Verification items for this drawing (mm, ordinates from the low corner). A direction names the side the tool comes from. Coordinates: 2 decimals unless noted, no trailing zeros. Order: outer loops, then holes, each group sorted by start corner. A loop starts at its lowest first (then second) coordinate and runs counter-clockwise, first axis right, second up. Notation, with made-up numbers: M 10,-25.5 L 22,-25.5 A7 ccw 22,-16.5 Z; hole C 60,55 d1. An arc over 180 degrees is marked long. Answer as a JSON object with one key per item and string values. Group by question number.
(1) Gauge pin test, flat ends, axial feed: pin 1 Ø5 at (y, z) = (11.5, 11.5) entering from -X; pin 2 Ø5 at (y, z) = (7.5, 28) entering from -X; pin 3 Ø3 at (y, z) = (9, 8.5) entering from +X; pin 4 Ø10 at (y, z) = (11.5, 12) entering from +X. Record the tip position at first contact, or that the pin passes through.
(2) Cross-section at D-D (z = 9.5). Enter the section's corners in (x, y), plus the area to 3 significant figures.
(3) Cross-section at C-C (x = 23). Enter the section's corners in (y, z), plus the area to 3 significant figures.
(4) Material ranges on line 1 (Z direction, x = 47, y = 4.75); line 2 (Z direction, x = 56.5, y = 14); line 3 (X direction, y = 1.75, z = 27.5) (1 decimal), recorded low to high.
(5) Access from +Z, -Z, +X, -X, +Y, -Y to the whole of each face (thin tool, end or side, straight path). Record for the marked faces 1, 2 and 3.
(6) Cross-section at B-B (y = 9.5). Enter the section's corners in (x, z), plus the area to 3 significant figures.
(7) Cross-section at A-A (x = 62). Enter the section's corners in (y, z).
(8) Mould release check, pull along Z, two halves, no side actions. Record for the marked faces 4, 5, 6 and 7: released by +Z, released by -Z, zero draft, split by the parting line, or undercut.
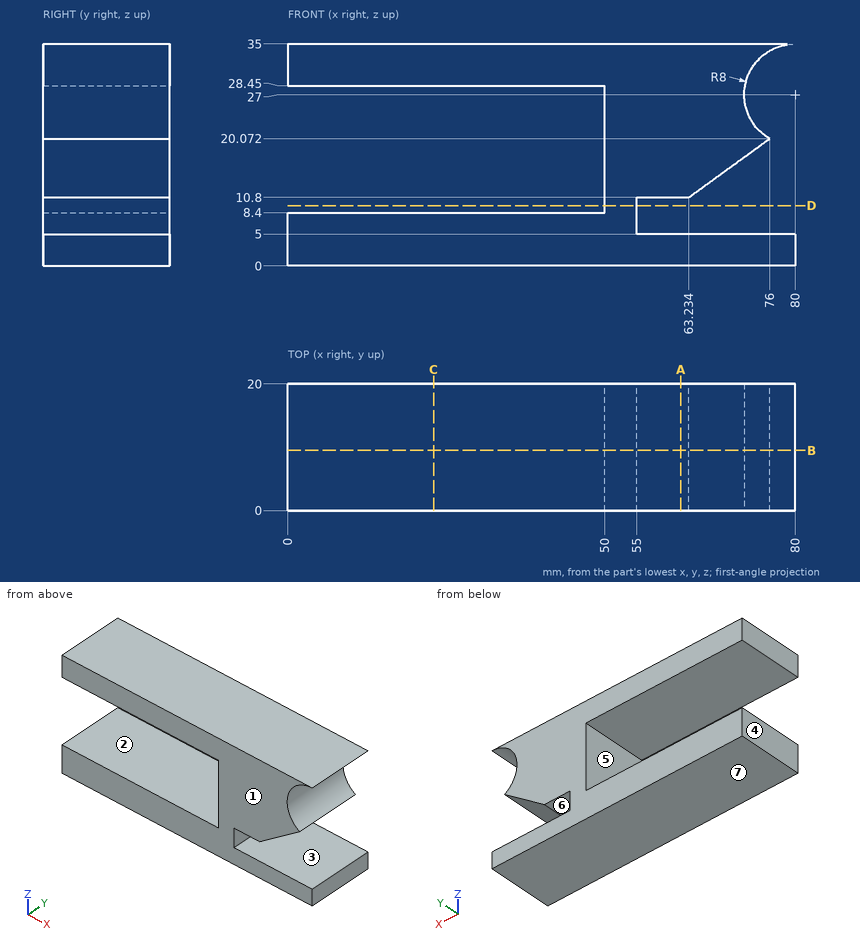
Taken from the geometry:
{
 "1": {"pin 1": "stops at x = 50", "pin 2": "stops at x = 0", "pin 3": "stops at x = 55", "pin 4": "stops at x = 71.77"},
 "2": {"outline": "M 50,0 L 55,0 L 55,20 L 50,20 Z", "area": "100 mm²"},
 "3": {"outline": "M 0,0 L 20,0 L 20,8.4 L 0,8.4 Z; M 0,28.45 L 20,28.45 L 20,35 L 0,35 Z", "area": "299 mm²"},
 "4": {"line 1": "z = 0 to 8.4, 28.45 to 35", "line 2": "z = 0 to 5, 10.8 to 35", "line 3": "x = 50 to 72"},
 "5": {"face 1": "+Z, -Z, +X, -X, -Y", "face 2": "-X, +Y, -Y", "face 3": "+X, +Y, -Y"},
 "6": {"outline": "M 0,0 L 80,0 L 80,5 L 55,5 L 55,10.8 L 63.23,10.8 L 76,20.07 A8 cw 80,35 L 0,35 L 0,28.45 L 50,28.45 L 50,8.4 L 0,8.4 Z", "area": "1,460 mm²"},
 "7": {"outline": "M 0,0 L 20,0 L 20,5 L 0,5 Z; M 0,10.8 L 20,10.8 L 20,35 L 0,35 Z"},
 "8": {"face 4": "zero draft", "face 5": "undercut", "face 6": "undercut", "face 7": "released by -Z"}
}
